Answer from the drawing. Dimensions are ordinates in mm from the lowest x, y and z of the part. Give positions to 0.01 mm unless a question says otherwise; leave off trailing zeros. Loops run counter-clockwise (first coordinate to the right, second up) from the corner with the lowest first, then second, coordinate; pieces in that order, holes last. Notation, with made-up numbers: (50.5, 0.25) - (73.5, 0.25) arc R20 ccw to (73.5, 7.25) - close; hole circle Ø2 at (64.25, 70). An arc over 180 degrees is marked (long way). Answer as CSV lines item,"result". Start each with the question number.
1) A cutting plane is placed at D-D (z = 8.5). Determine the outline of the cut face in (x, y), and give its area (3 significant figures).
2) A cutting plane is placed at A-A (z = 76.5). Determine the outline of the cut face in (x, y).
3) A cutting plane is placed at C-C (x = 49). Determine the outline of the cut face in (y, z).
4) A cutting plane is placed at B-B (y = 3.35). Determine the outline of the cut face in (x, z), and give its area (3 significant figures).
5) Flat-ended cylindrical pins translate along their axes: pin 1 (1.2 mm diameter, centred on x = 46.5, y = 1, fed in from -Z); pin 2 (2 mm diameter, centred on y = 1, z = 12.5, fed in from -X); pin 3 (2 mm diameter, centred on y = 3, z = 77.5, fed in from -X). Find the tip coordinate at first contact, or state that the pin passes through.
6) Find the intervals of material crossed by line 1 along Z through (x, y) = (38.5, 2.6); line 2 along X through (y, z) = (2.65, 5); line 3 along X through (y, z) = (0.25, 6), in increasing order.
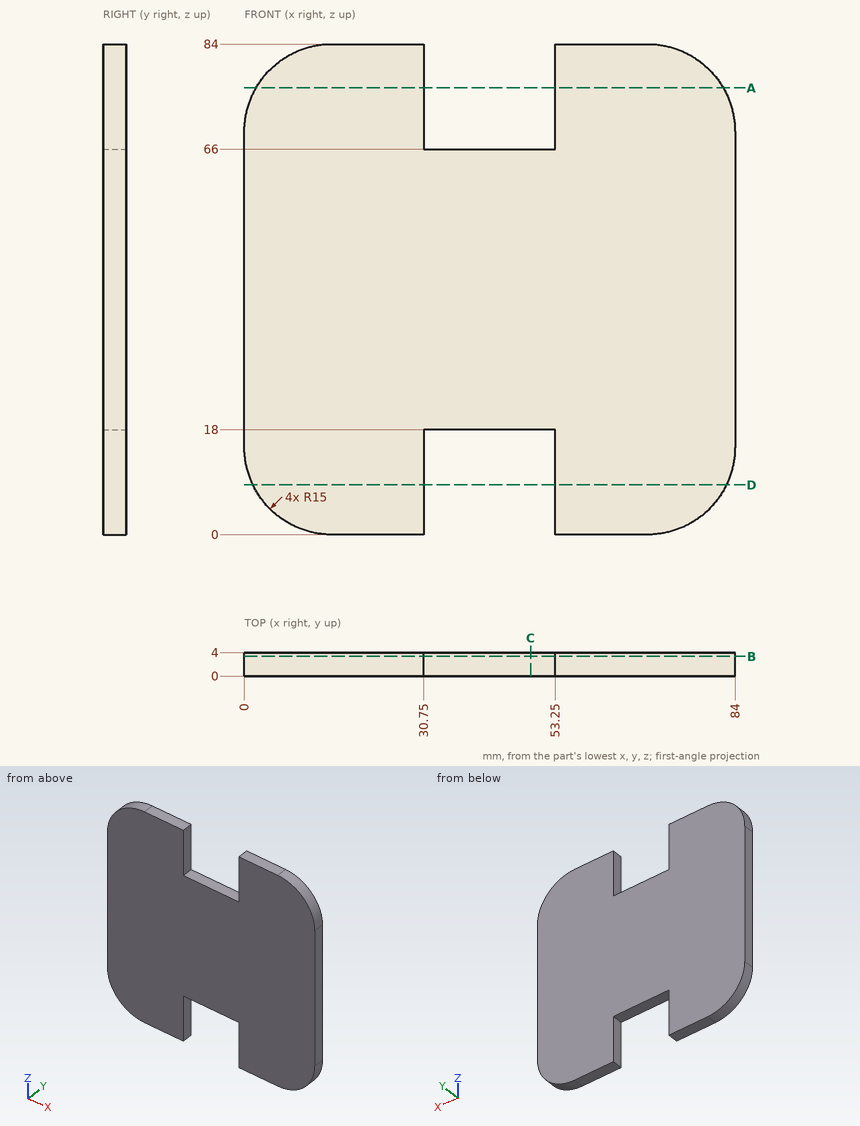
Ans:
1,outline,"(1.48, 0) - (30.75, 0) - (30.75, 4) - (1.48, 4) - close; (53.25, 0) - (82.52, 0) - (82.52, 4) - (53.25, 4) - close"
1,area,"234 mm2"
2,outline,"(2.01, 0) - (30.75, 0) - (30.75, 4) - (2.01, 4) - close; (53.25, 0) - (81.99, 0) - (81.99, 4) - (53.25, 4) - close"
3,outline,"(0, 18) - (4, 18) - (4, 66) - (0, 66) - close"
4,outline,"(0, 15) arc R15 ccw to (15, 0) - (30.75, 0) - (30.75, 18) - (53.25, 18) - (53.25, 0) - (69, 0) arc R15 ccw to (84, 15) - (84, 69) arc R15 ccw to (69, 84) - (53.25, 84) - (53.25, 66) - (30.75, 66) - (30.75, 84) - (15, 84) arc R15 ccw to (0, 69) - close"
4,area,"6,050 mm2"
5,pin 1,"z = 18"
5,pin 2,"x = 0.08"
5,pin 3,"x = 2.01"
6,line 1,"18 to 66"
6,line 2,"3.82 to 30.75, 53.25 to 80.18"
6,line 3,"3 to 30.75, 53.25 to 81"
